from build123d import *

# Parameters (mm, degrees)
RESSALTO_EXTRUS_O1_DEPTH = 8
ESBO_O3_R                = 2
CORTE_EXTRUS_O1_DEPTH    = 13.125139244


with BuildPart() as part:
    # Esboço2 → Ressalto-extrusão1 (new body)
    with BuildSketch(Plane.XY):
        with BuildLine():
            Line((42.125139244, 205.781065113), (30.947664044, 205.195278459))
            ThreePointArc((30.947664044, 205.195278459), (30.274625629, 204.8850035), (30, 204.196648925))
            Line((30, 204.196648925), (30, 200.565481301))
            ThreePointArc((30, 200.565481301), (30.274625629, 199.877126725), (30.947664044, 199.566851766))
            Line((30.947664044, 199.566851766), (42.125139244, 198.981065113))
            Line((42.125139244, 198.981065113), (42.125139244, 205.781065113))
        make_face()
    extrude(amount=-RESSALTO_EXTRUS_O1_DEPTH)

    # Esboço3 → Corte-extrusão1 (cut, through all)
    with BuildSketch(Plane(origin=(42.125139244, 0, 0), x_dir=(0, 0, -1), z_dir=(1, 0, 0))):
        with Locations((4, 202.381065113)):
            Circle(ESBO_O3_R)
    extrude(amount=-CORTE_EXTRUS_O1_DEPTH, mode=Mode.SUBTRACT)


solid = part.part
Input: part model. Units: mm. Frame: model coordinates. Give positions to 0.01 mm unless a question says otherwise; leave off trailing zeros. Write each loop counter-clockwise with the first axis right and the second up, starting at its lowest first coordinate (ties: lowest second). Pieces come first, ordered by that corner, then holes. Notation, with made-up numbers: M -35.75,35.5 L -22.75,35.5 A18 ccw -22.75,45.5 Z; hole C 42.25,31 d8. An arc over 180 degrees is marked long. Use one line per item in the form item = value.
1. Cut plane B-B on y = 203.5. Return loops of the section in (x, z).
Outcome:
outline = M 30,-8 L 42.13,-8 L 42.13,-5.66 L 30,-5.66 Z; M 30,-2.34 L 42.13,-2.34 L 42.13,0 L 30,0 Z
2. First-contact query: P1, Ø3, axis at y = 202.38, z = -4, coming from the -X side; P2, Ø2, axis at x = 34, y = 201.5, coming from the +Z side; P3, Ø1, axis at x = 33.5, z = -7, coming from the +Y side; P4, Ø1.5, axis at x = 40, z = -5, coming from the -Y side. Flat tips, straight axial feed; report the tip coordinate or a pass-through.
Outcome:
P1 = through
P2 = 0
P3 = 205.36
P4 = 199.05
3. Mould query, pull axis Y, two halves, no side actions, for faces 1 (the face through (30.28, 204.89, -3.94)), 2 (the face through (30, 202, -7)), 3 (the face through (36.147, 200.607, -4.923)). Classes: released by +Y, released by -Y, zero draft, split by the parting line, or undercut.
Outcome:
face_1 = released by +Y
face_2 = zero draft
face_3 = undercut
4. Cut plane C-C on x = 37.5. Return loops of the section in (y, z), and give its area (3 significant figures).
Outcome:
outline = M 199.22,-8 L 205.54,-8 L 205.54,0 L 199.22,0 Z; hole C 202.38,-4 d4
area = 38.0 mm²
5. Cut plane D-D on z = -6.25. Return loops of the section in (x, y), and give its area (3 significant figures).
Outcome:
outline = M 30,200.57 A1 ccw 30.95,199.57 L 42.13,198.98 L 42.13,205.78 L 30.95,205.2 A1 ccw 30,204.2 Z
area = 74.4 mm²
6. Ray query, L1, parallel to Z at x = 40.5, y = 202.5; L2, parallel to Y at x = 35.75, z = -3; L3, parallel to Z at x = 31, y = 201.75. Return the intervals inside material, ascending.
Outcome:
L1 = -8 to -6, -2 to 0
L2 = 199.32 to 200.65, 204.11 to 205.45
L3 = -8 to -5.9, -2.1 to 0
7. Cut plane A-A on z = -4.25. Return loops of the section in (x, y), and give its area (3 significant figures).
Outcome:
outline = M 30.01,200.4 A1 ccw 30.95,199.57 L 42.13,198.98 L 42.13,200.4 Z; M 30.01,204.37 L 42.13,204.37 L 42.13,205.78 L 30.95,205.2 A1 ccw Z
area = 26.2 mm²
